Read the model definition and answer for the solid it produces. Units are mm, in the model's axes. Coordinates: 2 decimals unless noted, no trailing zeros. Loops run counter-clockwise (first coordinate to the right, second up) from the corner with the lowest first, then second, coordinate; pieces in that order, holes last. Notation, with made-up numbers: (11, 52.5) -> (50, 52.5) arc R21 cw to (50, 75.5) -> close; hole circle Ø4 at (-12, 51.25). An arc over 180 degrees is marked (long way). Answer as a JSON object with one key per item and string values. Group by question number.
1) Section B-B, the plane z = 1 is taken. Count the separate pieces of the cut face and the enclosed holes in it, plus the area to 3 significant figures.
2) Consider probe 1 along X at (y, z) = (8.5, 0.05) (3 decimals); probe 2 along X at (y, z) = (-1.5, 1) (3 decimals); probe 3 along Y at (x, z) = (0, 0.75). Determine where each line is inside the solid, lowest interval first. Write a range as [from, to].
3) Determine the mould class of faces 1 (the face through (-30.627, 0.954, 0.022)), 2 (the face through (79, 0, 1.588)) for opening direction Y: released by +Y, released by -Y, zero draft, split by the parting line, or undercut.
4) Flat-ended cylindrical pins translate along their axes: P1, Ø7, axis at x = 203.61, y = 8.99, coming from the -Z side; P2, Ø5.5, axis at x = 151.07, y = 0, coming from the +Z side; P3, Ø7, axis at x = 165.67, y = 8.99, coming from the +Z side. Find the tip coordinate at first contact, or state that the pin passes through.
5) Section A-A, the plane x = 0 is taken. Give the vertices of the cut face in (y, z).
from build123d import *

# Parameters (mm, degrees)
SKETCH1_R                                         = 8.334375
BOSS_EXTRUDE1_DEPTH                               = 1.5875
F_6_CLEARANCE_HOLE3_D                             = 4.3053
CUT_EXTRUDE1_DEPTH                                = 4.175
CHAMFER1_SIZE                                     = 3.81
CSK_FOR_6_FLAT_HEAD_MACHINE_SCREW_100_D           = 4.3053
CSK_FOR_6_FLAT_HEAD_MACHINE_SCREW_100_CSINK_D     = 7.0866
CSK_FOR_6_FLAT_HEAD_MACHINE_SCREW_100_CSINK_ANGLE = 100
SKETCH14_W                                        = 50.8
SKETCH14_H                                        = 38.1
BOSS_EXTRUDE2_DEPTH                               = 3.175
CHAMFER2_SIZE                                     = 2.54
F_1_4_0_25_DIAMETER_HOLE1_D                       = 6.35


with BuildPart() as part:
    # Sketch1 → Boss-Extrude1 (new body, symmetric)
    with BuildSketch(Plane.XY):
        Polygon((0, 19.05), (-28.575, 19.05), (-28.575, -19.05), (0, -19.05), (247.281942035, -19.05), (254, 19.05), align=None)
        Circle(SKETCH1_R, mode=Mode.SUBTRACT)
    extrude(amount=BOSS_EXTRUDE1_DEPTH, both=True)

    # #6 Clearance Hole3 (through all)
    with Locations(Plane.XY.offset(1.5875)):
        with Locations((229.388701471, 8.923791784), (229.282371239, -11.346798968), (203.503161764, -11.143926969), (203.608782335, 8.991375351), (165.672159691, 8.991375351), (165.672159691, -11.143926969), (151.067159691, 0)):
            Hole(F_6_CLEARANCE_HOLE3_D / 2)

    # Sketch9 → Cut-Extrude1 (cut, through all)
    with BuildSketch(Plane.XY.offset(1.5875)):
        Polygon((254, 19.05), (247.281942035, -19.05), (237.352085197, -19.05), (237.352085197, 19.05), align=None)
    extrude(amount=-CUT_EXTRUDE1_DEPTH, mode=Mode.SUBTRACT)

    # Chamfer1
    chamfer1_edges = [part.edges().sort_by_distance(p)[0] for p in [
        (-28.575, -19.05, 0),
        (-28.575, 19.05, 0),
        (237.352085197, 19.05, 0),
        (237.352085197, -19.05, 0),
    ]]
    chamfer(chamfer1_edges, length=CHAMFER1_SIZE)

    # CSK for #6 Flat Head Machine Screw (100)2 (through all)
    with Locations(Plane.XY.offset(1.5875)):
        with Locations((203.608782335, 8.991375351), (203.503161764, -11.143926969), (229.282371239, -11.346798968), (229.388701471, 8.923791784), (165.672159691, 8.991375351), (165.672159691, -11.143926969), (151.067159691, 0)):
            CounterSinkHole(CSK_FOR_6_FLAT_HEAD_MACHINE_SCREW_100_D / 2, CSK_FOR_6_FLAT_HEAD_MACHINE_SCREW_100_CSINK_D / 2, counter_sink_angle=CSK_FOR_6_FLAT_HEAD_MACHINE_SCREW_100_CSINK_ANGLE)

    # Sketch14 → Boss-Extrude2 (add, through all)
    with BuildSketch(Plane.XY.offset(1.5875)):
        with Locations((-50.165, 0)):
            Rectangle(SKETCH14_W, SKETCH14_H)
    extrude(amount=-BOSS_EXTRUDE2_DEPTH)

    # Chamfer2
    chamfer2_edges = [part.edges().sort_by_distance(p)[0] for p in [
        (-75.565, -19.05, 0),
        (-75.565, 19.05, 0),
    ]]
    chamfer(chamfer2_edges, length=CHAMFER2_SIZE)

    # Sketch16 → CSK for #10 Flat Head Machine Screw (100)1 (revolve, cut)
    with BuildSketch(Plane(origin=(-65.405, 0, -1.5875), x_dir=(0, 1, 0), z_dir=(1, 0, 0))):
        Polygon((0, 0), (0, 3.175), (2.8067, 3.175), (2.8067, 1.747676712), (4.8895, 0), align=None)
    revolve(axis=Axis((-65.405, 0, -7.9375), (0, 0, 1)), mode=Mode.SUBTRACT)

    # 1/4 (0.25) Diameter Hole1 (through all)
    with Locations(Plane(origin=(0, 0, -1.5875), x_dir=(-1, 0, 0), z_dir=(0, 0, -1))):
        with Locations((33.655, 0)):
            Hole(F_1_4_0_25_DIAMETER_HOLE1_D / 2)


solid = part.part
Determined:
{
 "1": {"separate pieces": "1", "enclosed holes": "10", "area": "11,400 mm²"},
 "2": {"probe 1": "[-75.565, 163.576], [167.768, 201.513], [205.705, 227.278], [231.499, 237.352]", "probe 2": "[-75.565, -67.777], [-63.033, -36.453], [-30.857, -8.198], [8.198, 148.652], [153.482, 237.352]", "probe 3": "[-19.05, -8.33], [8.33, 19.05]"},
 "3": {"face 1": "undercut", "face 2": "zero draft"},
 "4": {"P1": "z = -1.59", "P2": "z = 0.92", "P3": "z = 1.55"},
 "5": {"outline": "(-19.05, -1.59) -> (-8.33, -1.59) -> (-8.33, 1.59) -> (-19.05, 1.59) -> close; (8.33, -1.59) -> (19.05, -1.59) -> (19.05, 1.59) -> (8.33, 1.59) -> close"}
}
